Build history of the part. All positions in model axes, mm. A direction names the side the tool comes from. Give positions to 0.01 mm unless a question says otherwise; leave off trailing zeros. Order: outer loops, then holes, each group sorted by start corner. A loop starts at its lowest first (then second) coordinate and runs counter-clockwise, first axis right, second up. Notation, with made-up numbers: M 29.5,-26.5 L 87.5,-26.5 A23 cw 87.5,10.5 Z; hole C 54,89.25 d1. An arc over 180 degrees is marked long. One line per item, written item: value. Start each with the question number.
from build123d import *

# Parameters (mm, degrees)
BOSS_EXTRUDE1_DEPTH = 76.2
CUT_EXTRUDE1_DEPTH  = 144.369655065
FILLET1_R           = 2.54


with BuildPart() as part:
    # Sketch2 → Boss-Extrude1 (new body)
    with BuildSketch(Plane.XY):
        Polygon((31.81322426, 23.302810647), (30.988, 24.061604353), (30.988, 22.40534), (112.268, 22.40534), (112.268, 23.302810647), align=None)
        with BuildLine():
            Line((30.988, 22.40534), (30.988, 24.061604353))
            Line((30.988, 24.061604353), (26.38332828, 28.2956))
            Line((26.38332828, 28.2956), (0, 28.2956))
            ThreePointArc((0, 28.2956), (-20.008010638, -20.008010638), (28.2956, 0))
            Line((28.2956, 0), (28.2956, 18.01114))
            Line((28.2956, 18.01114), (112.268, 18.01114))
            Line((112.268, 18.01114), (112.268, 19.23034))
            Line((112.268, 19.23034), (30.988, 19.23034))
            Line((30.988, 19.23034), (27.0764, 19.23034))
            Line((27.0764, 19.23034), (27.0764, 0))
            ThreePointArc((27.0764, 0), (-19.14590605, -19.14590605), (0, 27.0764))
            Line((0, 27.0764), (25.908, 27.0764))
            Line((25.908, 27.0764), (30.988, 22.40534))
        make_face()
    extrude(amount=BOSS_EXTRUDE1_DEPTH)

    # Sketch3 → Cut-Extrude1 (cut, through all)
    with BuildSketch(Plane.XZ.offset(-18.01114)):
        Polygon((112.268, 76.2), (30.988, 0), (112.268, 0), align=None)
    extrude(amount=-CUT_EXTRUDE1_DEPTH, mode=Mode.SUBTRACT)

    # Fillet1
    fillet1_edges = [part.edges().sort_by_distance(p)[0] for p in [
        (112.268, 18.62074, 76.2),
        (30.988, 18.62074, 0),
        (30.988, 23.233472177, 0),
        (112.268, 22.854075323, 76.2),
    ]]
    fillet(fillet1_edges, radius=FILLET1_R)


solid = part.part
1) Tool access for faces 5 (the flat face through (61, 22.405, 46)), 6 (the flat face through (27.076, 10, 38)), 7 (the flat face through (28.296, 9, 38)): list every direction of +Z, -Z, +X, -X, +Y, -Y with a clear straight run to the whole face (end or side of a thin tool).
2) Slice it at D-D (z = 61.5). List the corners of the cut face in (x, y), plus the area to 3 significant figures.
3) Pull direction X, two halves, no side cores. Call faces 1 (the cylindrical face through (-18.5, -19.77, 37.57)), 2 (the flat face through (13, 27.076, 38)), 3 (the cylindrical face through (108.222, 22.86, 74.554)), 4 (the flat face through (-10.1, 25.3, 0)): pulls with the +X half, pulls with the -X half, needs draft (parallel to the pull), parting line crosses it, or undercut.
4) Drop flat-ended pins along their axis: P1, Ø5, axis at x = 49.5, z = 25, coming from the -Y side; P2, Ø15.5, axis at y = 14, z = 19, coming from the -X side; P3, Ø6, axis at x = 29.5, z = 21, coming from the +Y side; P4, Ø23, axis at x = 82.5, z = 27, coming from the -Y side. Give the stop position or say it passes through.
5) Slice it at C-C (z = 9). List the corners of the cut face in (x, y).
6) Drill centre lines: line 1 (Y direction, x = 35.5, z = 63.5); line 2 (Y direction, x = 0.5, z = 10); line 3 (X direction, y = -16.5, z = 69.5). Where is each one in solid material? Low to high.
7) Slice it at A-A (x = 47.5). List the corners of the cut face in (y, z), plus the area to 3 significant figures.
8) Slice it at B-B (y = -6). List the corners of the cut face in (x, z).
Results list:
1. face 5: +Z, -Z, +X
1. face 6: +Z, -Z
1. face 7: +Z, -Z, +X, -Y
2. outline: M 0,27.08 L 25.91,27.08 L 30.99,22.41 L 96.59,22.41 L 96.59,23.3 L 31.81,23.3 L 26.38,28.3 L 0,28.3 A28.3 ccw long 28.3,0 L 28.3,18.01 L 96.59,18.01 L 96.59,19.23 L 27.08,19.23 L 27.08,0 A27.08 cw long Z
2. area: 365 mm²
3. face 1: undercut
3. face 2: undercut
3. face 3: pulls with the +X half
3. face 4: needs draft
4. P1: stops at y = 18.01
4. P2: stops at x = -27.6
4. P3: stops at y = 28.19
4. P4: passes through
5. outline: M 0,27.08 L 25.91,27.08 L 30.99,22.41 L 40.59,22.41 L 40.59,23.3 L 31.81,23.3 L 26.38,28.3 L 0,28.3 A28.3 ccw long 28.3,0 L 28.3,18.01 L 40.59,18.01 L 40.59,19.23 L 27.08,19.23 L 27.08,0 A27.08 cw long Z
6. line 1: y = 18.01 to 19.23, 22.41 to 23.3
6. line 2: y = -28.29 to -27.07, 27.08 to 28.3
6. line 3: x = -22.99 to -21.47, 21.47 to 22.99
7. outline: M 18.01,15.48 L 19.23,15.48 L 19.23,76.2 L 18.01,76.2 Z; M 22.41,15.48 L 23.3,15.48 L 23.3,76.2 L 22.41,76.2 Z
7. area: 129 mm²
8. outline: M -27.65,0 L -26.4,0 L -26.4,76.2 L -27.65,76.2 Z; M 26.4,0 L 27.65,0 L 27.65,76.2 L 26.4,76.2 Z
